```python
from build123d import *

# Parameters (mm, degrees)
BOSS_EXTRUDE1_DEPTH = 50
SKETCH4_R           = 3.15
CUT_EXTRUDE1_DEPTH  = 10
SKETCH10_R          = 3.425
CUT_EXTRUDE5_DEPTH  = 10
SKETCH12_W          = 80
SKETCH12_H          = 5
BOSS_EXTRUDE2_DEPTH = 50


with BuildPart() as part:
    # Sketch2 → Boss-Extrude1 (new body)
    with BuildSketch(Plane.XY):
        Polygon((-40.869025982, 215.979452737), (-40.869025982, 0), (59.130974018, 0), (59.130974018, 175), (46.975601581, 243.936542711), align=None)
        Polygon((0, 10), (49.130974018, 10), (49.130974018, 87.5), (49.130974018, 175), (39.440396213, 229.957997724), (6.085967265, 220.428944505), (-30.869025982, 207.731789579), (-30.869025982, 107.989726368), (-30.869025982, 10), align=None, mode=Mode.SUBTRACT)
    extrude(amount=BOSS_EXTRUDE1_DEPTH)

    # Sketch4 → Cut-Extrude1 (cut)
    with BuildSketch(Plane(origin=(87.274719522, 15.388887785, 0), x_dir=(0, 0, -1), z_dir=(0.984807753, 0.173648178, 0))):
        with Locations((-25, 202.690370895)):
            Circle(SKETCH4_R)
    extrude(amount=-CUT_EXTRUDE1_DEPTH, mode=Mode.SUBTRACT)

    # Sketch10 → Cut-Extrude5 (cut)
    with BuildSketch(Plane(origin=(0, 10, 0), x_dir=(1, 0, 0), z_dir=(0, 1, 0))):
        with Locations((-5.851287133, -25)):
            Circle(SKETCH10_R)
        with Locations((24.130974018, -25)):
            Circle(SKETCH10_R)
    extrude(amount=-CUT_EXTRUDE5_DEPTH, mode=Mode.SUBTRACT)

    # Sketch12 → Boss-Extrude2 (add)
    with BuildSketch(Plane.XY.offset(50)):
        with Locations((9.130974018, 172.5)):
            Rectangle(SKETCH12_W, SKETCH12_H)
        with Locations((9.130974018, 90)):
            Rectangle(SKETCH12_W, SKETCH12_H)
    extrude(amount=-BOSS_EXTRUDE2_DEPTH)


solid = part.part
```
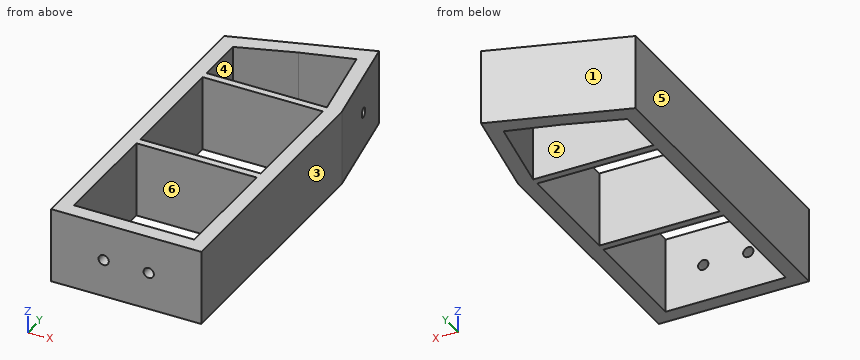
Work out the finished part from the listing and answer in its coordinate system (mm). Face numbers are marked on the shaded views. A direction names the side the tool comes from. Give positions to 0.01 mm unless a question says otherwise; leave off trailing zeros. Write each loop counter-clockwise with the first axis right and the second up, starting at its lowest first coordinate (ties: lowest second). Pieces come first, ordered by that corner, then holes. Notation, with made-up numbers: (-22.5, 3.25) -> (-5.5, 3.25) arc R18 ccw to (-5.5, 33.25) -> close; hole circle Ø4 at (43, 46.5). An arc over 180 degrees is marked (long way). Write item = value, one per line.
Q1. For a pull along X with two mould halves and no side action, classify the marked faces 3, 4, 5 and 6 as pulls with the +X half, pulls with the -X half, needs draft (parallel to the pull), parting line crosses it, or undercut.
Computed values:
face_3 = pulls with the +X half
face_4 = undercut
face_5 = pulls with the -X half
face_6 = undercut
Q2. Section B-B on z = 34 is taken. Determine the outline of the cut face in (x, y).
Computed values:
outline = (-40.87, 0) -> (59.13, 0) -> (59.13, 175) -> (46.98, 243.94) -> (-40.87, 215.98) -> close; hole (-30.87, 10) -> (49.13, 10) -> (49.13, 87.5) -> (-30.87, 87.5) -> close; hole (-30.87, 92.5) -> (49.13, 92.5) -> (49.13, 170) -> (-30.87, 170) -> close; hole (-30.87, 175) -> (49.13, 175) -> (39.44, 229.96) -> (6.09, 220.43) -> (-30.87, 207.73) -> close
Q3. A tool of negligible diameter and unlimited length cuts with its end or side. For the marked faces 1 and 2, from which of +Z, -Z, +X, -X, +Y, -Y can it reach the whole face along a straight path? Write none if from no direction.
Computed values:
face_1 = +Z, -Z, -X, +Y
face_2 = +Z, -Z
Q4. Section C-C on x = 31.5 is taken. Determine the outline of the cut face in (y, z), and give its area (3 significant figures).
Computed values:
outline = (0, 0) -> (10, 0) -> (10, 50) -> (0, 50) -> close; (87.5, 0) -> (92.5, 0) -> (92.5, 50) -> (87.5, 50) -> close; (170, 0) -> (175, 0) -> (175, 50) -> (170, 50) -> close; (227.69, 0) -> (239.01, 0) -> (239.01, 50) -> (227.69, 50) -> close
area = 1,570 mm^2
Q5. Flat-ended cylindrical pins translate along their axes: pin 1 Ø8 at (x, z) = (24.13, 25) entering from +Y; pin 2 Ø5.5 at (x, z) = (-5.85, 25) entering from +Y. Find the tip coordinate at first contact, or state that the pin passes through.
Computed values:
pin_1 = 237.94
pin_2 = 228
Q6. Consider line 1 along X through (y, z) = (6, 25); line 2 along X through (y, z) = (12, 46.5); line 3 along Y through (x, z) = (-4, 16.5). Determine where each line is inside the solid, lowest interval first.
Computed values:
line_1 = -40.87 to -9.28, -2.43 to 20.71, 27.56 to 59.13
line_2 = -40.87 to -30.87, 49.13 to 59.13
line_3 = 0 to 10, 87.5 to 92.5, 170 to 175, 216.96 to 227.71
Q7. Section A-A on y = 35.5 is taken. Determine the outline of the cut face in (x, z), and give its area (3 significant figures).
Computed values:
outline = (-40.87, 0) -> (-30.87, 0) -> (-30.87, 50) -> (-40.87, 50) -> close; (49.13, 0) -> (59.13, 0) -> (59.13, 50) -> (49.13, 50) -> close
area = 1,000 mm^2
